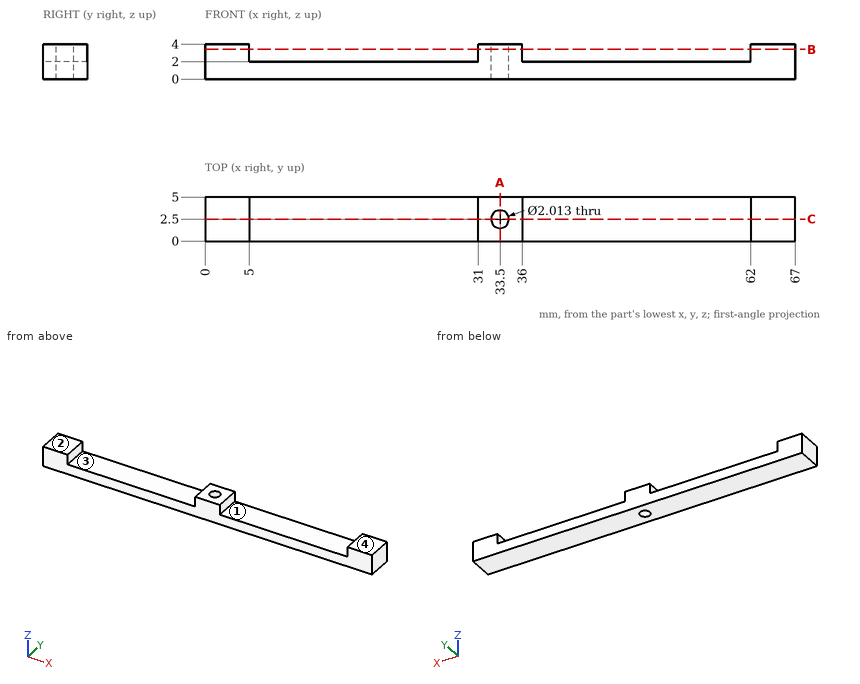
Part print with two shaded views. Sizes in mm from the minimum x, y, z corner. A direction names the side the tool comes from. Coordinates: 2 decimals unless noted, no trailing zeros. Write each loop counter-clockwise with the first axis right and the second up, starting at its lowest first coordinate (ties: lowest second). Pieces come first, ordered by that corner, then holes. Notation, with made-up numbers: (75, 62) - (110, 62) arc R32 cw to (110, 98) - close; hole circle Ø5 at (-13.5, 42.5). An arc over 180 degrees is marked (long way). One line per item, written item: value. Start each with the question number.
1. Slice it at C-C (y = 2.5). Write the cut outline in (x, z).
2. Flat gauge pin, fed straight in: pin 1 (1.5 mm diameter, centred on x = 45.5, y = 2, fed in from +Z). Where does the tip first touch, or does it go through?
3. Mould opens along X. For the marked faces 1 and 2 say: released by +X, released by -X, zero draft, split by the parting line, or undercut.
4. Tool access for the marked faces 3 and 4: list every direction of +Z, -Z, +X, -X, +Y, -Y with a clear straight run to the whole face (end or side of a thin tool).
5. Slice it at A-A (x = 33.5). Write the cut outline in (y, z).
6. Probe line 1 (X direction, y = 0.8, z = 3.3); line 2 (X direction, y = 2.5, z = 2.55); line 3 (Y direction, x = 33.5, z = 1.9). List the from-to ranges inside material, lowest first. Write a range as from..to.
7. Slice it at B-B (z = 3.4). Write the cut outline in (x, y), plus the area to 3 significant figures.
Answers below:
1. outline: (0, 0) - (32.49, 0) - (32.49, 4) - (31, 4) - (31, 2) - (5, 2) - (5, 4) - (0, 4) - close; (34.51, 0) - (67, 0) - (67, 4) - (62, 4) - (62, 2) - (36, 2) - (36, 4) - (34.51, 4) - close
2. pin 1: stops at z = 2
3. face 1: undercut
3. face 2: zero draft
4. face 3: +Z, +Y, -Y
4. face 4: +Z, +X, -X, +Y, -Y
5. outline: (0, 0) - (1.49, 0) - (1.49, 4) - (0, 4) - close; (3.51, 0) - (5, 0) - (5, 4) - (3.51, 4) - close
6. line 1: x = 0..5, 31..36, 62..67
6. line 2: x = 0..5, 31..32.49, 34.51..36, 62..67
6. line 3: y = 0..1.49, 3.51..5
7. outline: (0, 0) - (5, 0) - (5, 5) - (0, 5) - close; (31, 0) - (36, 0) - (36, 5) - (31, 5) - close; (62, 0) - (67, 0) - (67, 5) - (62, 5) - close; hole circle Ø2.01 at (33.5, 2.5)
7. area: 71.8 mm^2
